Work out the finished part from the listing and answer in its coordinate system (mm). A direction names the side the tool comes from. Coordinates: 2 decimals unless noted, no trailing zeros. Write each loop counter-clockwise with the first axis right and the second up, starting at its lowest first coordinate (ties: lowest second). Pieces come first, ordered by that corner, then holes. Notation, with made-up numbers: (-39.5, 63) - (-18.5, 63) arc R14 ccw to (-18.5, 69) - close; hole circle Ø10 at (27.25, -33.5). An arc over 180 degrees is marked (long way). Use one line per item in the form item = value. Start each with the question number.
Item 1: A cutting plane is placed at C-C (y = 27). Write down the section's boundary in (x, z).
Item 2: For faces 1 (the flat face through (0, 44.45, -15)), 2 (the flat face through (0, 31.75, -17)), 3 (the cylindrical face through (9.12, 22.719, -9.945)), 4 (the flat face through (0, 30.162, -20)), determine the directions among +Z, -Z, +X, -X, +Y, -Y from which every point of the face is accessible in a straight line to the end or side of a thin tool.
Item 3: Determine the mould class of faces 5 (the flat face through (0, 18.256, -17)), 6 (the flat face through (0, 1.588, 0)), 7 (the flat face through (0, 10, -20.638)) for opening direction Y: released by +Y, released by -Y, zero draft, split by the parting line, or undercut.
Item 4: A cutting plane is placed at A-A (z = -18). Write down the section's boundary in (x, y).
Item 5: Given pin 1 (6.5 mm diameter, centred on x = -6, y = 25.5, fed in from -Z); pin 2 (3 mm diameter, centred on x = 7, y = 38, fed in from +Z); pin 3 (8 mm diameter, centred on x = -2, z = -4, fed in from +Y), each flat-ended and moving along its own axis, determine where each tip first touches the part or whether it passes through.
Item 6: Consider probe 1 along Z at (x, y) = (0, 19); probe 2 along Z at (x, y) = (0, 24); probe 3 along Y at (x, z) = (-5, -16.5). Determine where each line is inside the solid, lowest interval first.
Item 7: A cutting plane is placed at D-D (z = 7). Write down the section's boundary in (x, y).
Item 8: A cutting plane is placed at B-B (x = 0). Write down the section's boundary in (y, z).
from build123d import *

# Parameters (mm, degrees)
SKETCH1_R           = 13.49375
BOSS_EXTRUDE1_DEPTH = 44.45
SKETCH2_R           = 15.08125
BOSS_EXTRUDE2_DEPTH = 1.5875
CUT_EXTRUDE1_DEPTH  = 58.545506449


with BuildPart() as part:
    # Sketch1 → Boss-Extrude1 (new body)
    with BuildSketch(Plane(origin=(0, 0, 0), x_dir=(1, 0, 0), z_dir=(0, 1, 0))):
        with BuildLine():
            Line((-15.08125, 0), (-15.08125, 20.6375))
            Line((-15.08125, 20.6375), (15.08125, 20.6375))
            Line((15.08125, 20.6375), (15.08125, 0))
            ThreePointArc((15.08125, 0), (0, -15.08125), (-15.08125, 0))
        make_face()
        with Locations(Location((0, 0, 0), (0, 0, 270))):
            Circle(SKETCH1_R, mode=Mode.SUBTRACT)
    extrude(amount=BOSS_EXTRUDE1_DEPTH)

    # Sketch2 → Boss-Extrude2 (add)
    with BuildSketch(Plane.XZ):
        Circle(SKETCH2_R)
    extrude(amount=-BOSS_EXTRUDE2_DEPTH)

    # Sketch3 → Cut-Extrude1 (cut, through all)
    with BuildSketch(Plane(origin=(15.08125, 0, 0), x_dir=(0, 0, -1), z_dir=(1, 0, 0))):
        Polygon((20.6375, 30.1625), (19.05, 30.1625), (19.05, 31.75), (15.08125, 31.75), (15.08125, 18.25625), (19.05, 18.25625), (19.05, 19.84375), (20.6375, 19.84375), align=None)
    extrude(amount=-CUT_EXTRUDE1_DEPTH, mode=Mode.SUBTRACT)


solid = part.part
Answer:
q1.outline = (-15.08, -15.08) - (15.08, -15.08) - (15.08, 0) arc R15.08 ccw to (-15.08, 0) - close; hole circle Ø26.99 at (0, 0)
q2.face_1 = +Z, -Z, +X, -X, +Y
q2.face_2 = +X, -X
q2.face_3 = +Y
q2.face_4 = -Z, +X, -X
q3.face_5 = undercut
q3.face_6 = released by +Y
q3.face_7 = zero draft
q4.outline = (-15.08, 0) - (15.08, 0) - (15.08, 18.26) - (-15.08, 18.26) - close; (-15.08, 31.75) - (15.08, 31.75) - (15.08, 44.45) - (-15.08, 44.45) - close
q5.pin_1 = -15.08
q5.pin_2 = 14.04
q5.pin_3 = 1.59
q6.probe_1 = -20.64 to -19.05, -15.08 to -13.49, 13.49 to 15.08
q6.probe_2 = -15.08 to -13.49, 13.49 to 15.08
q6.probe_3 = 0 to 18.26, 31.75 to 44.45
q7.outline = (-13.36, 0) - (13.36, 0) - (13.36, 44.45) - (11.54, 44.45) - (11.54, 1.59) - (-11.54, 1.59) - (-11.54, 44.45) - (-13.36, 44.45) - close
q8.outline = (0, -20.64) - (19.84, -20.64) - (19.84, -19.05) - (18.26, -19.05) - (18.26, -15.08) - (31.75, -15.08) - (31.75, -19.05) - (30.16, -19.05) - (30.16, -20.64) - (44.45, -20.64) - (44.45, -13.49) - (1.59, -13.49) - (1.59, 13.49) - (44.45, 13.49) - (44.45, 15.08) - (0, 15.08) - close
